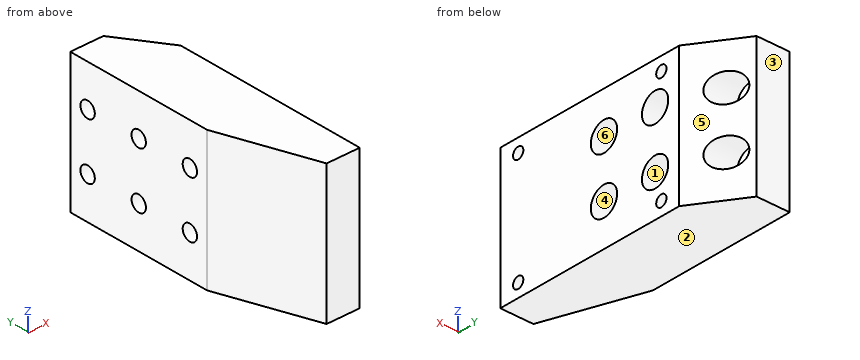
```python
from build123d import *

# Parameters (mm, degrees)
BOSS_EXTRUDE1_DEPTH         = 63
SKETCH3_R                   = 3.5687
CUT_EXTRUDE1_DEPTH          = 63
SKETCH4_R                   = 6.5405
CUT_EXTRUDE2_DEPTH          = 20
F_1_4_20_TAPPED_HOLE1_D     = 5.1054
F_1_4_20_TAPPED_HOLE1_DEPTH = 10
F_1_4_20_TAPPED_HOLE1_TIP   = 1.533816902


with BuildPart() as part:
    # Sketch1 → Boss-Extrude1 (new body)
    with BuildSketch(Plane.XY):
        Polygon((-38.72257574, 45.396234333), (-38.72257574, -22.603765667), (-23.72257574, -65.503765667), (-8.72257574, -65.503765667), (-8.72257574, 23.396234333), (-23.72257574, 45.396234333), align=None)
    extrude(amount=BOSS_EXTRUDE1_DEPTH)

    # Sketch3 → Cut-Extrude1 (cut)
    with BuildSketch(Plane.ZY.offset(38.72257574)):
        with Locations((18.8, 36.796234333)):
            Circle(SKETCH3_R)
        with Locations((44.2, 36.796234333)):
            Circle(SKETCH3_R)
        with Locations((18.8, 11.396234333)):
            Circle(SKETCH3_R)
        with Locations((44.2, 11.396234333)):
            Circle(SKETCH3_R)
        with Locations((18.8, -14.003765667)):
            Circle(SKETCH3_R)
        with Locations((44.2, -14.003765667)):
            Circle(SKETCH3_R)
    extrude(amount=-CUT_EXTRUDE1_DEPTH, mode=Mode.SUBTRACT)

    # Sketch4 → Cut-Extrude2 (cut)
    with BuildSketch(Plane(origin=(-8.72257574, 0, 0), x_dir=(0, 0, -1), z_dir=(1, 0, 0))):
        with Locations((-44.2, -14.003765667)):
            Circle(SKETCH4_R)
        with Locations((-18.8, -14.003765667)):
            Circle(SKETCH4_R)
        with Locations((-18.8, 11.396234333)):
            Circle(SKETCH4_R)
        with Locations((-44.2, 36.796234333)):
            Circle(SKETCH4_R)
        with Locations((-18.8, 36.796234333)):
            Circle(SKETCH4_R)
        with Locations((-44.2, 11.396234333)):
            Circle(SKETCH4_R)
    extrude(amount=-CUT_EXTRUDE2_DEPTH, mode=Mode.SUBTRACT)

    # 1/4-20 Tapped Hole1
    with Locations(Plane(origin=(-8.72257574, 0, 0), x_dir=(0, 0, -1), z_dir=(1, 0, 0))):
        with Locations((-56.9, 14.506234333), (-6.1, 14.506234333), (-56.9, -56.613765667), (-6.1, -56.613765667)):
            Hole(F_1_4_20_TAPPED_HOLE1_D / 2, depth=F_1_4_20_TAPPED_HOLE1_DEPTH)
            with Locations((0, 0, -(F_1_4_20_TAPPED_HOLE1_DEPTH + F_1_4_20_TAPPED_HOLE1_TIP / 2))):  # 118° drill point
                Cone(0, F_1_4_20_TAPPED_HOLE1_D / 2, F_1_4_20_TAPPED_HOLE1_TIP, mode=Mode.SUBTRACT)


solid = part.part
```
Can you work these out from the model? Positions are in its coordinate system, mm. Face numbers are marked on the shaded views. A direction names the side the tool comes from. Round coordinates to 2 decimals unless told otherwise and drop trailing zeros. Order: outer loops, then holes, each group sorted by start corner. A loop starts at its lowest first (then second) coordinate and runs counter-clockwise, first axis right, second up.
(1) If I drill on L1, parallel to Y at x = -19.75, z = 44.2; L2, parallel to Z at x = -23, y = 35; L3, parallel to Z at x = -35.5, y = 10, over which ranges is the centre line in solid material (lowest first)?
Results are:
L1: y = -65.5 to -20.54, -7.46 to 4.86, 17.94 to 30.26
L2: z = 0 to 12.51, 25.09 to 37.91, 50.49 to 63
L3: z = 0 to 15.52, 22.08 to 40.92, 47.48 to 63
(2) On a 3-axis mill with a long thin cutter (end or side, diameter ignored), from which of +Z, -Z, +X, -X, +Y, -Y can I reach the whole of each face in a straight line? I mean the marked faces 5 and 6. Say none if no direction works.
Results are:
face 5: +Z, -Z, +X, +Y
face 6: +X
(3) We'd pull the mould along Z, two halves only. Please class the marked faces 1, 2, 3 and 4: +Z half, -Z half, draft (parallel to the pull), parting line (faces both ways), or undercut.
Results are:
face 1: undercut
face 2: -Z half
face 3: draft
face 4: undercut
(4) I'm going to push flat-ended pins straight in: pin 1 (6 mm diameter, centred on y = -56.61, z = 56.9, fed in from -X); pin 2 (12 mm diameter, centred on y = 36.8, z = 18.8, fed in from +X); pin 3 (6.5 mm diameter, centred on y = -14, z = 44.2, fed in from -X); pin 4 (14.5 mm diameter, centred on y = 37, z = 42, fed in from +X). Where does each tip first touch, or does it pass through?
Results are:
pin 1: stops at x = -27.88
pin 2: stops at x = -28.72
pin 3: passes through
pin 4: stops at x = -13.05
(5) If we section it at C-C (z = 30): Please give me the cut outline in (x, y), plus the area to 3 significant figures.
Results are:
outline: (-38.72, -22.6) - (-23.72, -65.5) - (-8.72, -65.5) - (-8.72, 23.4) - (-23.72, 45.4) - (-38.72, 45.4) - close
area: 2,840 mm2
(6) If we section it at A-A (z = 18.8): Count the separate pieces of the cut face and the enclosed holes in it, plus the area to 3 significant figures.
Results are:
separate pieces: 4
enclosed holes: 0
area: 1,960 mm2
(7) If we section it at B-B (y = 39): Please give me the cut outline in (x, z), plus the area to 3 significant figures.
Results are:
outline: (-38.72, 0) - (-19.36, 0) - (-19.36, 12.64) - (-28.72, 12.64) - (-28.72, 15.99) - (-38.72, 15.99) - close; (-38.72, 21.61) - (-28.72, 21.61) - (-28.72, 24.96) - (-19.36, 24.96) - (-19.36, 38.04) - (-28.72, 38.04) - (-28.72, 41.39) - (-38.72, 41.39) - close; (-38.72, 47.01) - (-28.72, 47.01) - (-28.72, 50.36) - (-19.36, 50.36) - (-19.36, 63) - (-38.72, 63) - close
area: 877 mm2
